Work out the finished part from the listing and answer in its coordinate system (mm). Coordinates: 2 decimals unless noted, no trailing zeros. Order: outer loops, then holes, each group sorted by start corner. A loop starts at its lowest first (then second) coordinate and runs counter-clockwise, first axis right, second up. Notation, with made-up numbers: M -26,-17.5 L -20,-17.5 A12 ccw -20,5.5 Z; hole C 47,-39.75 d11. An arc over 180 degrees is marked long. Answer in a Markdown table with one row per item. Add a question column.
Item 1: The part is cut by section C-C (y = 640). Write down the section's boundary in (x, z).
Item 2: The part is cut by section D-D (x = 360). Write down the section's boundary in (y, z).
Item 3: The mould has two halves that part along X. Classify faces 1 (the face through (161, 355, 40)), 2 (the face through (163.041, 405.932, 19.72)), 3 (the face through (372.418, 659.478, 20.28)), 4 (the face through (0, 345, 20)): released by +X, released by -X, zero draft, split by the parting line, or undercut.
Item 4: The part is cut by section A-A (y = 350). Write down the section's boundary in (x, z), then the cut area to 3 significant figures.
Item 5: Consider line 1 (Y direction, x = 360, z = 20); line 2 (Y direction, x = 258, z = 19); line 3 (X direction, y = 625, z = 8). Determine where each line is inside the solid, lowest interval first. Write a range as from..to.
Item 6: Flat-ended cylindrical pins translate along their axes: pin 1 Ø9.5 at (x, y) = (258, 302) entering from -Z; pin 2 Ø3 at (x, z) = (183, 20) entering from -Y. Find the tip coordinate at first contact, or state that the pin passes through.
Item 7: The part is cut by section B-B (x = 210). Write down the section's boundary in (y, z), then the cut area to 3 significant figures.
from build123d import *

# Parameters (mm, degrees)
SKETCH_1_W             = 420
SKETCH_1_H             = 700
EXTRUDE_1_DEPTH        = 40
SKETCH_2_R             = 23.1
CUT_EXTRUDE_1_DEPTH    = 818.312669668
SKETCH_3_R             = 26
CUT_EXTRUDE_2_DEPTH    = 818.312669668
M18X2_0_1_D            = 16
CHAMFER_1_SIZE         = 4
HOLE_WIZARD_M4_1_D     = 3.3
HOLE_WIZARD_M4_1_DEPTH = 10.1
HOLE_WIZARD_M4_1_TIP   = 0.991420021


with BuildPart() as part:
    # 草图1 → 凸台-拉伸1 (new body)
    with BuildSketch(Plane.XY):
        with Locations((210, 350)):
            Rectangle(SKETCH_1_W, SKETCH_1_H)
    extrude(amount=EXTRUDE_1_DEPTH)

    # 草图2 → 切除-拉伸1 (cut, through all)
    with BuildSketch(Plane.XY.offset(40)):
        with Locations((60, 60)):
            Circle(SKETCH_2_R)
        with Locations((360, 60)):
            Circle(SKETCH_2_R)
        with Locations((360, 640)):
            Circle(SKETCH_2_R)
        with Locations((60, 640)):
            Circle(SKETCH_2_R)
    extrude(amount=-CUT_EXTRUDE_1_DEPTH, mode=Mode.SUBTRACT)

    # 草图3 → 切除-拉伸2 (cut, through all)
    with BuildSketch(Plane.XY.offset(40)):
        with Locations((210, 350)):
            Circle(SKETCH_3_R)
    extrude(amount=-CUT_EXTRUDE_2_DEPTH, mode=Mode.SUBTRACT)

    # M18x2.0 螺纹孔1 (through all)
    with Locations(Plane.XY.offset(40)):
        with Locations((162, 398), (258, 398), (258, 302), (162, 302)):
            Hole(M18X2_0_1_D / 2)

    # 倒角1
    chamfer_1_edges = [part.edges().sort_by_distance(p)[0] for p in [
        (420, 350, 40),
        (210, 700, 40),
        (0, 350, 40),
        (210, 700, 0),
        (420, 350, 0),
        (210, 0, 0),
        (0, 350, 0),
        (210, 0, 40),
        (0, 700, 20),
        (420, 700, 20),
        (420, 0, 20),
        (0, 0, 20),
    ]]
    chamfer(chamfer_1_edges, length=CHAMFER_1_SIZE)

    # M4 螺纹孔1
    with Locations(Plane(origin=(0, 0, 0), x_dir=(-1, 0, 0), z_dir=(0, -1, 0))):
        with Locations((-237, -20), (-183, -20)):
            Hole(HOLE_WIZARD_M4_1_D / 2, depth=HOLE_WIZARD_M4_1_DEPTH)
            with Locations((0, 0, -(HOLE_WIZARD_M4_1_DEPTH + HOLE_WIZARD_M4_1_TIP / 2))):  # 118° drill point
                Cone(0, HOLE_WIZARD_M4_1_D / 2, HOLE_WIZARD_M4_1_TIP, mode=Mode.SUBTRACT)


solid = part.part
Reply:
| question | item | result |
|---|---|---|
| 1 | outline | M 0,4 L 4,0 L 36.9,0 L 36.9,40 L 4,40 L 0,36 Z; M 83.1,0 L 336.9,0 L 336.9,40 L 83.1,40 Z; M 383.1,0 L 416,0 L 420,4 L 420,36 L 416,40 L 383.1,40 Z |
| 2 | outline | M 0,4 L 4,0 L 36.9,0 L 36.9,40 L 4,40 L 0,36 Z; M 83.1,0 L 616.9,0 L 616.9,40 L 83.1,40 Z; M 663.1,0 L 696,0 L 700,4 L 700,36 L 696,40 L 663.1,40 Z |
| 3 | face 1 | zero draft |
| 3 | face 2 | undercut |
| 3 | face 3 | undercut |
| 3 | face 4 | released by -X |
| 4 | outline | M 0,4 L 4,0 L 184,0 L 184,40 L 4,40 L 0,36 Z; M 236,0 L 416,0 L 420,4 L 420,36 L 416,40 L 236,40 Z |
| 4 | area | 14,700 mm2 |
| 5 | line 1 | y = 0..36.9, 83.1..616.9, 663.1..700 |
| 5 | line 2 | y = 0..294, 310..390, 406..700 |
| 5 | line 3 | x = 0..42.43, 77.57..342.43, 377.57..420 |
| 6 | pin 1 | passes through |
| 6 | pin 2 | stops at y = 10.19 |
| 7 | outline | M 0,4 L 4,0 L 324,0 L 324,40 L 4,40 L 0,36 Z; M 376,0 L 696,0 L 700,4 L 700,36 L 696,40 L 376,40 Z |
| 7 | area | 25,900 mm2 |
